Input: part model. Units: mm. Frame: model coordinates. A direction names the side the tool comes from. Round coordinates to 2 decimals unless told otherwise and drop trailing zeros. Loops run counter-clockwise (first coordinate to the right, second up) from the corner with the lowest first, then second, coordinate; pieces in that order, holes last. Notation, with made-up numbers: M -24.75,33 L -11.75,33 A25 ccw -11.75,57 Z; hole C 58.5,-8.5 d6. An arc over 180 degrees is marked long. Use one line per item in the form item = value. Start each with the question number.
Q1. Ray query, line 1 along Y through (x, z) = (-12, 0.35); line 2 along Z through (x, y) = (-3, 7.75); line 3 along Y through (x, z) = (3, -3). Return the intervals inside material, ascending.
Q2. Section query C-C, the plane x = 12. Output: boundary loops of the cut face in (y, z), and give its area (3 significant figures).
Q3. Mould query, pull axis X, two halves, no side actions, for faces 1 (the cylindrical face through (-13, -12, 1)), 2 (the flat face through (4.75, 12, 2)), 3 (the flat face through (0, 13, 2)). Classes: pulls with the +X half, pulls with the -X half, needs draft (parallel to the pull), parting line crosses it, or undercut.
Q4. Section query B-B, the plane z = 1.75. Output: boundary loops of the cut face in (x, y), and give its area (3 significant figures).
Q5. Section query D-D, the plane y = -12. Output: boundary loops of the cut face in (x, z).
Q6. Access query for faces 4 (the flat face through (0, 0, 2.8)), 5 (the flat face through (-0.2, 7.816, -0.5)), 6 (the flat face through (0, -8, 0)). Directions: +Z, -Z, +X, -X, +Y, -Y. A direction counts if a zero-diameter tool reaches every point of the face in a straight line with its end or side. Return the directions, or none.
Q7. First-contact query: P1, Ø0.5, axis at x = 5.5, z = 2, coming from the +Y side; P2, Ø6, axis at y = 8.5, z = -6, coming from the +X side; P3, Ø1.6, axis at x = -12, y = 12, coming from the +Z side; P4, Ø3, axis at x = 1, y = 5.5, coming from the -Z side. Flat tips, straight axial feed; report the tip coordinate or a pass-through.
Q8. Section query A-A, the plane y = 12. Output: boundary loops of the cut face in (x, z).
```python
from build123d import *

# Parameters (mm, degrees)
F0_W          = 28
F0_H          = 4.5
F0_R          = 1
F0_W_2        = 9.5
F0_H_2        = 2
F0_H_3        = 1.684464
F0_H_4        = 4
F0_H_5        = 10
F0_H_6        = 7.815536
F1_DEPTH      = 1.25
F2_DEPTH      = 3.75
F2_DEPTH_BACK = 8.5
F3_DEPTH      = 1
F4_DEPTH      = 2.8


with BuildPart() as f1:
    # F0 (on Top) → F1 (new body)
    with BuildSketch(Plane.XY):
        with Locations((0, 11.75)):
            Rectangle(F0_W, F0_H)
        with Locations((-12, 12)):
            Circle(F0_R, mode=Mode.SUBTRACT)
        with Locations((0, 12)):
            Rectangle(F0_W_2, F0_H_2, mode=Mode.SUBTRACT)
        with Locations((12, 12)):
            Circle(F0_R, mode=Mode.SUBTRACT)
        with Locations((0, 12)):
            Rectangle(F0_W_2, F0_H_2)
        with Locations((0, 8.657768)):
            Rectangle(F0_W, F0_H_3)
        with Locations((0, -12)):
            Rectangle(F0_W, F0_H_4)
        with Locations((-12, -12)):
            Circle(F0_R, mode=Mode.SUBTRACT)
        with Locations((12, -12)):
            Circle(F0_R, mode=Mode.SUBTRACT)
        with Locations((0, 2.815536)):
            Rectangle(F0_W, F0_H_5)
        with Locations((0, -6.092232)):
            Rectangle(F0_W, F0_H_6)
    extrude(amount=F1_DEPTH)

    # F0 (on Top) → F2 (join, two sides)
    with BuildSketch(Plane.XY) as f2_sk:
        with Locations((0, 12)):
            Rectangle(F0_W_2, F0_H_2)
    extrude(amount=F2_DEPTH)
    extrude(f2_sk.sketch, amount=-F2_DEPTH_BACK)

    # F0 (on Top) → F3 (join)
    with BuildSketch(Plane.XY):
        with Locations((0, 2.815536)):
            Rectangle(F0_W, F0_H_5)
    extrude(amount=-F3_DEPTH)

    # F0 (on Top) → F4 (join)
    with BuildSketch(Plane.XY):
        with Locations((0, 2.815536)):
            Rectangle(F0_W, F0_H_5)
        with Locations((0, -6.092232)):
            Rectangle(F0_W, F0_H_6)
        with Locations((0, 8.657768)):
            Rectangle(F0_W, F0_H_3)
    extrude(amount=F4_DEPTH)


solid = f1.part
```
Results found:
q1.line_1 = -14 to -13, -11 to 11, 13 to 14
q1.line_2 = -1 to 2.8
q1.line_3 = 11 to 13
q2.outline = M -14,0 L -13,0 L -13,1.25 L -14,1.25 Z; M -11,0 L -2.18,0 L -2.18,-1 L 7.82,-1 L 7.82,0 L 11,0 L 11,1.25 L 9.5,1.25 L 9.5,2.8 L -10,2.8 L -10,1.25 L -11,1.25 Z; M 13,0 L 14,0 L 14,1.25 L 13,1.25 Z
q2.area = 70.2 mm²
q3.face_1 = undercut
q3.face_2 = pulls with the +X half
q3.face_3 = needs draft
q4.outline = M -14,-10 L 14,-10 L 14,9.5 L -14,9.5 Z; M -4.75,11 L 4.75,11 L 4.75,13 L -4.75,13 Z
q4.area = 565 mm²
q5.outline = M -14,0 L -13,0 L -13,1.25 L -14,1.25 Z; M -11,0 L 11,0 L 11,1.25 L -11,1.25 Z; M 13,0 L 14,0 L 14,1.25 L 13,1.25 Z
q6.face_4 = +Z, +X, -X, -Y
q6.face_5 = -Z, +X, -X
q6.face_6 = -Z, +X, -X, -Y
q7.P1 = 9.5
q7.P2 = 4.75
q7.P3 = through
q7.P4 = -1
q8.outline = M -14,0 L -13,0 L -13,1.25 L -14,1.25 Z; M -11,0 L -4.75,0 L -4.75,-8.5 L 4.75,-8.5 L 4.75,0 L 11,0 L 11,1.25 L 4.75,1.25 L 4.75,3.75 L -4.75,3.75 L -4.75,1.25 L -11,1.25 Z; M 13,0 L 14,0 L 14,1.25 L 13,1.25 Z
